```python
from build123d import *

# Parameters (mm, degrees)
F0_W     = 66
F0_H     = 66
F0_W_2   = 8
F0_H_2   = 55
F1_DEPTH = 2
F0_W_3   = 14
F0_H_3   = 10.5
F0_H_4   = 11.5
F2_DEPTH = 6
F3_DEPTH = 10
F0_W_4   = 4.0717534721
F0_H_5   = 7.087867707
F0_R     = 1.3859466119
F4_DEPTH = 3
F0_W_5   = 6.9370614365
F5_DEPTH = 5
F6_DEPTH = 2


with BuildPart() as f1:
    # F0 (on Top) → F1 (new body)
    with BuildSketch(Plane.XY):
        with Locations((33, 33)):
            Rectangle(F0_W, F0_H)
        Polygon((21.7376640153, 17.1879483869), (14.8006025788, 17.1879483869), (14.8006025788, 24.275816094), (21.7376640153, 24.275816094), (25.8094174874, 24.275816094), (25.8094174874, 17.1879483869), align=None, mode=Mode.SUBTRACT)
        Polygon((21.6838878947, 27.1878037923), (14.7468264583, 27.1878037923), (14.7468264583, 34.2756714994), (21.6838878947, 34.2756714994), (25.7556413668, 34.2756714994), (25.7556413668, 27.1878037923), align=None, mode=Mode.SUBTRACT)
        with Locations((6, 33)):
            Rectangle(F0_W_2, F0_H_2, mode=Mode.SUBTRACT)
        Polygon((21.6301117742, 37.1876591977), (14.6930503377, 37.1876591977), (14.6930503377, 44.2755269048), (21.6301117742, 44.2755269048), (25.7018652463, 44.2755269048), (25.7018652463, 37.1876591977), align=None, mode=Mode.SUBTRACT)
        Polygon((21.5763356537, 47.1875146031), (14.6392742172, 47.1875146031), (14.6392742172, 54.2753823102), (21.5763356537, 54.2753823102), (25.6480891258, 54.2753823102), (25.6480891258, 47.1875146031), align=None, mode=Mode.SUBTRACT)
        Polygon((48.5562719405, 45.5), (48.5562719405, 56), (62.5562719405, 56), (62.5562719405, 45.5), (62.5562719405, 44.5), (62.5562719405, 34), (62.5562719405, 33), (62.5562719405, 22.5), (62.5562719405, 21.5), (62.5562719405, 10), (48.5562719405, 10), (48.5562719405, 21.5), (48.5562719405, 22.5), (48.5562719405, 33), (48.5562719405, 34), (48.5562719405, 44.5), align=None, mode=Mode.SUBTRACT)
    extrude(amount=F1_DEPTH)

    # F0 (on Top) → F2 (join)
    with BuildSketch(Plane.XY):
        with Locations((55.5562719405, 50.75)):
            Rectangle(F0_W_3, F0_H_3)
        with Locations((55.5562719405, 39.25)):
            Rectangle(F0_W_3, F0_H_3)
        with Locations((55.5562719405, 27.75)):
            Rectangle(F0_W_3, F0_H_3)
        with Locations((55.5562719405, 15.75)):
            Rectangle(F0_W_3, F0_H_4)
    extrude(amount=F2_DEPTH)

    # F0 (on Top) → F3 (join)
    with BuildSketch(Plane.XY):
        with Locations((6, 33)):
            Rectangle(F0_W_2, F0_H_2)
    extrude(amount=F3_DEPTH)

    # F0 (on Top) → F4 (join)
    with BuildSketch(Plane.XY):
        with Locations((23.6122123897, 50.7314484566)):
            Rectangle(F0_W_4, F0_H_5)
        with Locations((23.7425714731, 50.7314484566)):
            Circle(F0_R, mode=Mode.SUBTRACT)
        with Locations((23.6659885103, 40.7315930512)):
            Rectangle(F0_W_4, F0_H_5)
        with Locations((23.7963475937, 40.7315930512)):
            Circle(F0_R, mode=Mode.SUBTRACT)
        with Locations((23.7197646308, 30.7317376458)):
            Rectangle(F0_W_4, F0_H_5)
        with Locations((23.8501237142, 30.7317376458)):
            Circle(F0_R, mode=Mode.SUBTRACT)
        with Locations((23.7735407513, 20.7318822405)):
            Rectangle(F0_W_4, F0_H_5)
        with Locations((23.9038998348, 20.7318822405)):
            Circle(F0_R, mode=Mode.SUBTRACT)
    extrude(amount=F4_DEPTH)

    # F0 (on Top) → F5 (join)
    with BuildSketch(Plane.XY):
        with Locations((18.1078049354, 50.7314484566)):
            Rectangle(F0_W_5, F0_H_5)
        with Locations((18.161581056, 40.7315930512)):
            Rectangle(F0_W_5, F0_H_5)
        with Locations((18.2153571765, 30.7317376458)):
            Rectangle(F0_W_5, F0_H_5)
        with Locations((18.2691332971, 20.7318822405)):
            Rectangle(F0_W_5, F0_H_5)
    extrude(amount=F5_DEPTH)

    # F0 (on Top) → F6 (join)
    with BuildSketch(Plane.XY):
        with Locations((23.7425714731, 50.7314484566)):
            Circle(F0_R)
        with Locations((23.7963475937, 40.7315930512)):
            Circle(F0_R)
        with Locations((23.8501237142, 30.7317376458)):
            Circle(F0_R)
        with Locations((23.9038998348, 20.7318822405)):
            Circle(F0_R)
    extrude(amount=F6_DEPTH)


solid = f1.part
```
For this review, take the finished solid that the model builds, in its own axes (mm). A direction names the side the tool comes from. Coordinates: 2 decimals unless noted, no trailing zeros. Write each loop counter-clockwise with the first axis right and the second up, starting at its lowest first coordinate (ties: lowest second). Pieces come first, ordered by that corner, then holes.
(1) Add section C-C on x = 17. Give the boundary of the cut face in (y, z), then the cut area to 3 significant figures.
(2) Tool access review of faces 5 (the face through (55, 44.5, 3)), 6 (the face through (18, 41, 5)), 7 (the face through (62.556, 16, 4)), 8 (the face through (24, 31, 2)): name each direction out of +Z, -Z, +X, -X, +Y, -Y from which nothing blocks a thin tool from reaching the whole face with its end or side.
(3) The part is to be moulded in two halves that separate along Y. For faces 1 (the face through (55, 10, 4)), 2 (the face through (19, 27.188, 3)), 3 (the face through (24, 51, 2)), 4 (the face through (66, 33, 1)), say which applies: +Y half, -Y half, draft (parallel to the pull), parting line (faces both ways), or undercut.
(4) Add section A-A on x = 60.5. Give the boundary of the cut face in (y, z), then the cut area to 3 significant figures.
(5) Wall thickness on probe 1 along X at (y, z) = (49.5, 4.25); probe 2 along Y at (x, z) = (53, 1.25); probe 3 along X at (y, z) = (48.5, 2.25): over which ranges is each line inside the solid? List them lowest first.
(6) Add section B-B on y = 12. Give the boundary of the cut face in (x, z), then the cut area to 3 significant figures.
(7) Add section D-D on z = 7.25. Give the boundary of the cut face in (x, y), then the cut area to 3 significant figures.
(8) For pin 1 Ø11.5 at (x, y) = (56.5, 52.5) entering from +Z; pin 2 Ø3 at (y, z) = (41, 4) entering from +X; pin 3 Ø1.5 at (x, z) = (20, 4) entering from +Y; pin 4 Ø1.5 at (x, z) = (27, 5) entering from +Y, all flat-tipped, find the tip position at first contact; note any pin that passes through.
Answer sheet:
1. outline: (0, 0) - (66, 0) - (66, 2) - (54.28, 2) - (54.28, 5) - (47.19, 5) - (47.19, 2) - (44.28, 2) - (44.28, 5) - (37.19, 5) - (37.19, 2) - (34.28, 2) - (34.28, 5) - (27.19, 5) - (27.19, 2) - (24.28, 2) - (24.28, 5) - (17.19, 5) - (17.19, 2) - (0, 2) - close
1. area: 217 mm2
2. face 5: +Z, -Z
2. face 6: +Z, +Y, -Y
2. face 7: +Z, +X, +Y, -Y
2. face 8: +Z
3. face 1: -Y half
3. face 2: undercut
3. face 3: undercut
3. face 4: draft
4. outline: (0, 0) - (21.5, 0) - (21.5, 6) - (10, 6) - (10, 2) - (0, 2) - close; (22.5, 0) - (33, 0) - (33, 6) - (22.5, 6) - close; (34, 0) - (44.5, 0) - (44.5, 6) - (34, 6) - close; (45.5, 0) - (66, 0) - (66, 2) - (56, 2) - (56, 6) - (45.5, 6) - close
4. area: 298 mm2
5. probe 1: x = 2 to 10, 14.64 to 21.58, 48.56 to 62.56
5. probe 2: y = 0 to 21.5, 22.5 to 33, 34 to 44.5, 45.5 to 66
5. probe 3: x = 2 to 10, 14.64 to 25.65, 48.56 to 62.56
6. outline: (0, 0) - (66, 0) - (66, 2) - (62.56, 2) - (62.56, 6) - (48.56, 6) - (48.56, 2) - (10, 2) - (10, 10) - (2, 10) - (2, 2) - (0, 2) - close
6. area: 252 mm2
7. outline: (2, 5.5) - (10, 5.5) - (10, 60.5) - (2, 60.5) - close
7. area: 440 mm2
8. pin 1: stops at z = 6
8. pin 2: stops at x = 62.56
8. pin 3: stops at y = 54.28
8. pin 4: passes through
